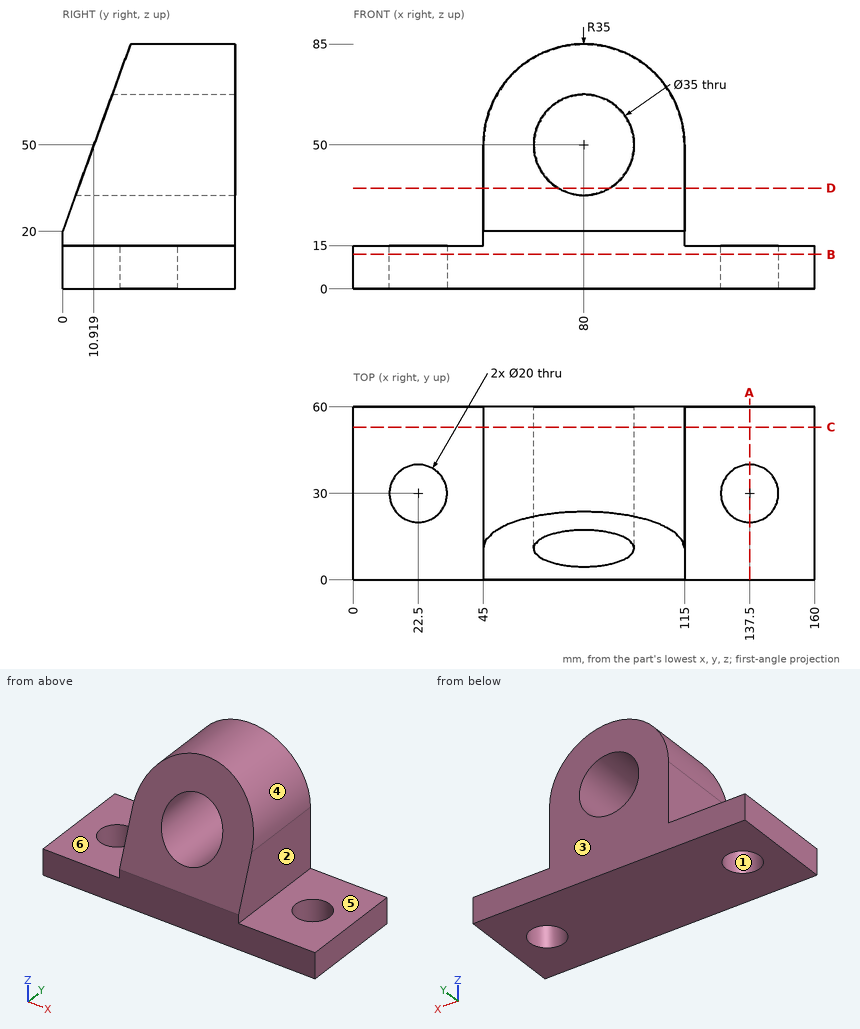
Could you check a few things on this drawing? It's one solid part, dimensions in mm from its lowest x, y, z. A direction names the side the tool comes from. Round coordinates to 2 decimals unless told otherwise and drop trailing zeros. Loops run counter-clockwise (first coordinate to the right, second up) from the corner with the lowest first, then second, coordinate; pieces in that order, holes last. Notation, with made-up numbers: (85, -38.75) -> (131, -38.75) arc R22 ccw to (131, -28.75) -> close; hole circle Ø9 at (34.25, -3). An arc over 180 degrees is marked (long way). Answer as CSV lines item,"result".
1. If I drill on L1, parallel to Z at x = 80, y = 35.5; L2, parallel to Y at x = 22.5, z = 9.75; L3, parallel to Z at x = 34, y = 33.5, over which ranges is the centre line in solid material (lowest first)?
Final values:
L1,"z = 0 to 32.5, 67.5 to 85"
L2,"y = 0 to 20, 40 to 60"
L3,"z = 0 to 15"
2. Which directions (+Z, -Z, +X, -X, +Y, -Y) give clear straight access to the entire face, cutting with the end or side of a thin tool? Please do the marked faces 4, 5 and 6.
Final values:
face 4,"+Z, +Y, -Y"
face 5,"+Z, +X, +Y, -Y"
face 6,"+Z, -X, +Y, -Y"
3. If we section it at A-A on x = 137.5: Please give me the cut outline in (y, z).
Final values:
outline,"(0, 0) -> (20, 0) -> (20, 15) -> (0, 15) -> close; (40, 0) -> (60, 0) -> (60, 15) -> (40, 15) -> close"
4. For pin 1 (1.5 mm diameter, centred on y = 50.5, z = 57.5, fed in from +X); pin 2 (12 mm diameter, centred on x = 99, y = 50.5, fed in from +Z); pin 3 (2 mm diameter, centred on y = 19.5, z = 68.5, fed in from -X); pin 4 (12 mm diameter, centred on x = 137.5, y = 30, fed in from -Z), each with a flat end and sliding along its axis, tell me the tip position at first contact or that it passes through.
Final values:
pin 1,"stops at x = 114.34"
pin 2,"stops at z = 82.5"
pin 3,"stops at x = 49.69"
pin 4,"passes through"
5. If we section it at C-C on y = 53: Please give me the cut outline in (x, z).
Final values:
outline,"(0, 0) -> (160, 0) -> (160, 15) -> (115, 15) -> (115, 50) arc R35 ccw to (45, 50) -> (45, 15) -> (0, 15) -> close; hole circle Ø35 at (80, 50)"
6. If we section it at B-B on z = 12: Please give me the cut outline in (x, y).
Final values:
outline,"(0, 0) -> (160, 0) -> (160, 60) -> (0, 60) -> close; hole circle Ø20 at (22.5, 30); hole circle Ø20 at (137.5, 30)"
7. If we section it at D-D on z = 35: Please give me the cut outline in (x, y).
Final values:
outline,"(45, 5.46) -> (70.99, 5.46) -> (70.99, 60) -> (45, 60) -> close; (89.01, 5.46) -> (115, 5.46) -> (115, 60) -> (89.01, 60) -> close"
8. Thinking about a two-plate mould opening in Y: for the marked faces 1, 2 and 3, which applies, released by +Y, released by -Y, zero draft, split by the parting line, or undercut?
Final values:
face 1,"undercut"
face 2,"zero draft"
face 3,"released by +Y"
